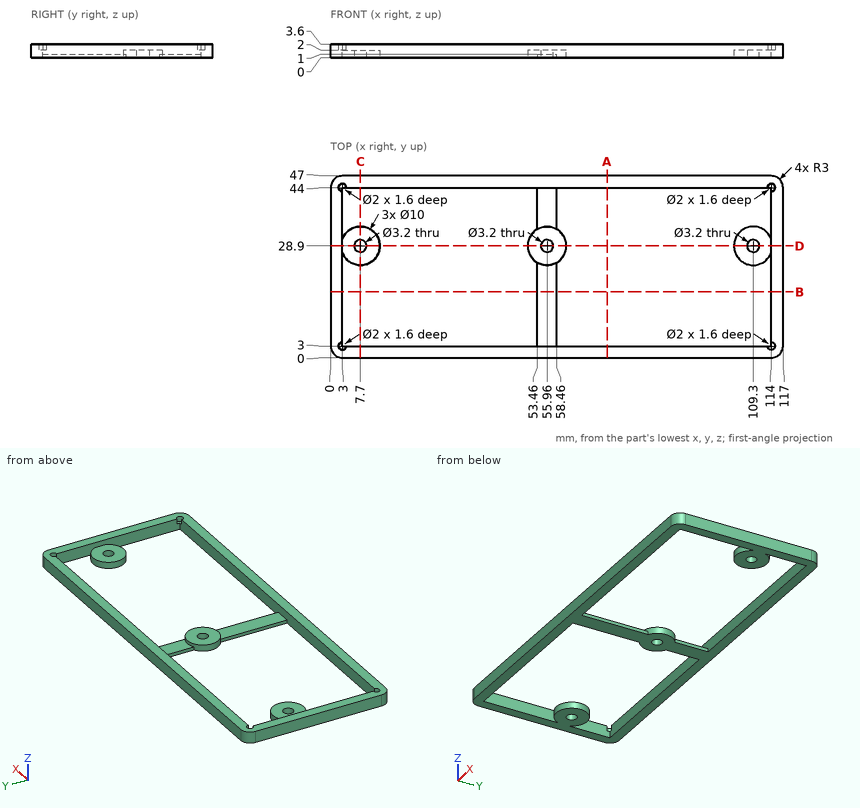
Could you check a few things on this drawing? It's one solid part, dimensions in mm from its lowest x, y, z. Coordinates: 2 decimals unless noted, no trailing zeros. Loops run counter-clockwise (first coordinate to the right, second up) from the corner with the lowest first, then second, coordinate; pieces in that order, holes last.
1. Imagine slicing it at B-B (y = 17). Please give me the cut outline in (x, z).
2. Imagine slicing it at D-D (y = 28.9). Please give me the cut outline in (x, z), and give its area (3 significant figures).
3. For P1, Ø0.6, axis at x = 3, y = 3, coming from the +Z side; P2, Ø2, axis at x = 114.5, y = 44.5, coming from the +Z side; P3, Ø2.5, axis at x = 55, y = 40.5, coming from the +Z side, each with a flat end and sliding along its axis, tell me the tip position at first contact or that it passes through.
4. I need wall thicknesses on L1, parallel to Y at x = 7.7, z = 1.05; L2, parallel to Y at x = 95, z = 2.1; L3, parallel to X at y = 10.5, z = 2.85. Which ranges of each line are inside material? Lowest first, please.
5. Imagine slicing it at C-C (x = 7.7). Please give me the cut outline in (y, z).
6. Imagine slicing it at A-A (x = 71.5). Please give me the cut outline in (y, z), and give its area (3 significant figures).
Computed values:
1. outline: (0, 0) - (3, 0) - (3, 3.6) - (0, 3.6) - close; (53.46, 0) - (58.46, 0) - (58.46, 1) - (53.46, 1) - close; (114, 0) - (117, 0) - (117, 3.6) - (114, 3.6) - close
2. outline: (0, 0) - (6.1, 0) - (6.1, 2) - (3, 2) - (3, 3.6) - (0, 3.6) - close; (9.3, 0) - (12.7, 0) - (12.7, 2) - (9.3, 2) - close; (50.96, 0) - (54.36, 0) - (54.36, 2) - (50.96, 2) - close; (57.56, 0) - (60.96, 0) - (60.96, 2) - (57.56, 2) - close; (104.3, 0) - (107.7, 0) - (107.7, 2) - (104.3, 2) - close; (110.9, 0) - (117, 0) - (117, 3.6) - (114, 3.6) - (114, 2) - (110.9, 2) - close
2. area: 61.2 mm2
3. P1: stops at z = 2
3. P2: stops at z = 3.6
3. P3: stops at z = 1
4. L1: y = 0 to 3, 23.9 to 27.3, 30.5 to 33.9, 44 to 47
4. L2: y = 0 to 3, 44 to 47
4. L3: x = 0 to 3, 114 to 117
5. outline: (0, 0) - (3, 0) - (3, 3.6) - (0, 3.6) - close; (23.9, 0) - (27.3, 0) - (27.3, 2) - (23.9, 2) - close; (30.5, 0) - (33.9, 0) - (33.9, 2) - (30.5, 2) - close; (44, 0) - (47, 0) - (47, 3.6) - (44, 3.6) - close
6. outline: (0, 0) - (3, 0) - (3, 3.6) - (0, 3.6) - close; (44, 0) - (47, 0) - (47, 3.6) - (44, 3.6) - close
6. area: 21.6 mm2
